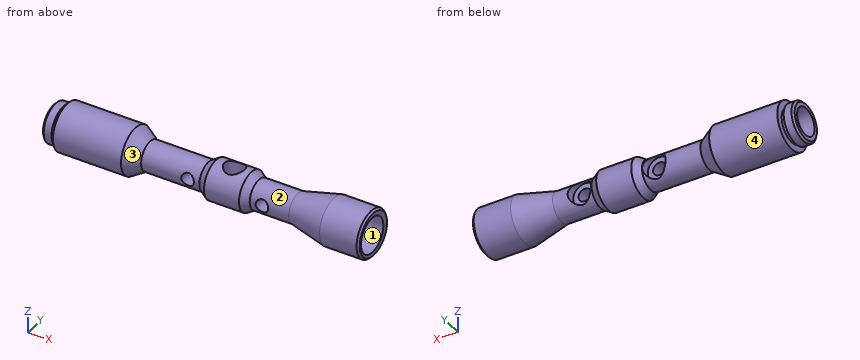
from build123d import *

# Parameters (mm, degrees)
HOLE_WIZARD_9_D            = 10
HOLE_WIZARD_9_DEPTH        = 50
HOLE_WIZARD_9_CBORE_D      = 14
HOLE_WIZARD_9_CBORE_DEPTH  = 20
HOLE_WIZARD_9_TIP          = 2.886751346
HOLE_WIZARD_M12_1_D        = 10.2
HOLE_WIZARD_M12_1_DEPTH    = 12
HOLE_WIZARD_M12_1_TIP      = 3.064389157
CHAMFER_1_SIZE             = 1
CHAMFER_2_SIZE             = 1
HOLE_WIZARD_12_D           = 10
HOLE_WIZARD_12_DEPTH       = 40
HOLE_WIZARD_12_CBORE_D     = 18
HOLE_WIZARD_12_CBORE_DEPTH = 20
HOLE_WIZARD_12_TIP         = 2.886751346
HOLE_WIZARD_14_D           = 6.5
HOLE_WIZARD_14_DEPTH       = 100
HOLE_WIZARD_14_CBORE_D     = 12
HOLE_WIZARD_14_CBORE_DEPTH = 4.5
HOLE_WIZARD_15_D           = 6.5
HOLE_WIZARD_15_DEPTH       = 100
HOLE_WIZARD_15_CBORE_D     = 12
HOLE_WIZARD_15_CBORE_DEPTH = 4.5


with BuildPart() as part:
    # 草图2 → 旋转2 (revolve)
    with BuildSketch(Plane.XY, mode=Mode.PRIVATE) as revolve_2_sk:
        Polygon((0, 10), (0, 0), (164, 0), (164, 12), (144, 12), (125.3, 7.582380862), (105.3, 7.582380862), (101.324359639, 10), (83.324359639, 10), (79.4, 7.5), (49.4, 7.5), (42, 12), (7, 12), (7, 8.5), (5, 8.5), (5, 10), align=None)
    revolve(revolve_2_sk.sketch.rotate(Axis((0, 0, 0), (1, 0, 0)), 180), axis=Axis((0, 0, 0), (1, 0, 0)))

    # 孔9
    with Locations(Plane.ZY):
        with Locations((0, 0)):
            CounterBoreHole(HOLE_WIZARD_9_D / 2, HOLE_WIZARD_9_CBORE_D / 2, HOLE_WIZARD_9_CBORE_DEPTH, depth=HOLE_WIZARD_9_DEPTH)
            with Locations((0, 0, -(HOLE_WIZARD_9_DEPTH + HOLE_WIZARD_9_TIP / 2))):  # 120° drill point
                Cone(0, HOLE_WIZARD_9_D / 2, HOLE_WIZARD_9_TIP, mode=Mode.SUBTRACT)

    # M12 螺纹孔1
    with Locations(Plane(origin=(92.712048687, 0.00356299, 9.999999365), x_dir=(0, 0.999999936526, -0.000356298984), z_dir=(0, 0.000356298984, 0.999999936526))):
        with Locations((0, 0)):
            Hole(HOLE_WIZARD_M12_1_D / 2, depth=HOLE_WIZARD_M12_1_DEPTH)
            with Locations((0, 0, -(HOLE_WIZARD_M12_1_DEPTH + HOLE_WIZARD_M12_1_TIP / 2))):  # 118° drill point
                Cone(0, HOLE_WIZARD_M12_1_D / 2, HOLE_WIZARD_M12_1_TIP, mode=Mode.SUBTRACT)

    # 倒角1
    chamfer_1_edges = [part.edges().sort_by_distance(p)[0] for p in [
        (164, 12, 0),
    ]]
    chamfer(chamfer_1_edges, length=CHAMFER_1_SIZE)

    # 倒角2
    chamfer_2_edges = [part.edges().sort_by_distance(p)[0] for p in [
        (0, 10, 0),
    ]]
    chamfer(chamfer_2_edges, length=CHAMFER_2_SIZE)

    # 孔12
    with Locations(Plane(origin=(164, 0, 0), x_dir=(0, 0, -1), z_dir=(1, 0, 0))):
        with Locations((-0.105297268, -0.976154466)):
            CounterBoreHole(HOLE_WIZARD_12_D / 2, HOLE_WIZARD_12_CBORE_D / 2, HOLE_WIZARD_12_CBORE_DEPTH, depth=HOLE_WIZARD_12_DEPTH)
            with Locations((0, 0, -(HOLE_WIZARD_12_DEPTH + HOLE_WIZARD_12_TIP / 2))):  # 120° drill point
                Cone(0, HOLE_WIZARD_12_D / 2, HOLE_WIZARD_12_TIP, mode=Mode.SUBTRACT)

    # 孔14
    with Locations(Plane(origin=(73.309592569, 7.499999992, 0.000348053), x_dir=(0, -4.6407092e-05, 0.999999998923), z_dir=(0, 0.999999998923, 4.6407092e-05))):
        with Locations((0, 0)):
            CounterBoreHole(HOLE_WIZARD_14_D / 2, HOLE_WIZARD_14_CBORE_D / 2, HOLE_WIZARD_14_CBORE_DEPTH, depth=HOLE_WIZARD_14_DEPTH)

    # 孔15
    with Locations(Plane(origin=(111.545186108, 7.582371257, 0.012068763), x_dir=(0, -0.001591685193, 0.999998733268), z_dir=(0, 0.999998733268, 0.001591685193))):
        with Locations((0, 0)):
            CounterBoreHole(HOLE_WIZARD_15_D / 2, HOLE_WIZARD_15_CBORE_D / 2, HOLE_WIZARD_15_CBORE_DEPTH, depth=HOLE_WIZARD_15_DEPTH)


solid = part.part
Build history of the part. All positions in model axes, mm. Face numbers are marked on the shaded views. A direction names the side the tool comes from. Coordinates: 2 decimals unless noted, no trailing zeros. Write each loop counter-clockwise with the first axis right and the second up, starting at its lowest first coordinate (ties: lowest second). Pieces come first, ordered by that corner, then holes. Notation, with made-up numbers: (-25.5, 54) -> (26.5, 54) arc R12 cw to (26.5, 77) -> close; hole circle Ø5 at (11.5, -35.75). An arc over 180 degrees is marked (long way). Use CSV: the item, a comma, the result in double quotes. Start each with the question number.
Q1. Pull direction X, two halves, no side cores. Call the marked faces 1 and 2: released by +X, released by -X, zero draft, split by the parting line, or undercut.
Q2. Cut at A-A, the plane x = 85. List the corners of the cut face in (y, z), then the cut area to 3 significant figures.
Q3. 3-axis set-ups, long thin cutter, end or side, ignore diameter. For the marked faces 3 and 4: which of +Z, -Z, +X, -X, +Y, -Y reach the whole face in a straight line?
Q4. Flat gauge pins, fed straight in: pin 1 Ø12 at (x, z) = (84.5, 0) entering from +Y; pin 2 Ø1.5 at (y, z) = (-3, -1.5) entering from +X; pin 3 Ø4 at (y, z) = (-1.5, -0.5) entering from +X; pin 4 Ø13 at (y, z) = (-0.98, 0.11) entering from -X. Where does each tip first touch, or does it go through?
Q5. Drill centre lines: probe 1 along Y at (x, z) = (97, 2); probe 2 along Z at (x, y) = (57.5, -0.5); probe 3 along X at (y, z) = (5.5, 0.75). Where is each one in solid material? Low to high.
Checked values:
1,face 1,"zero draft"
1,face 2,"undercut"
2,outline,"circle Ø20 at (0, 0)"
2,area,"314 mm²"
3,face 3,"none"
3,face 4,"+X, -X"
4,pin 1,"stops at y = 10"
4,pin 2,"stops at x = 123.04"
4,pin 3,"stops at x = 122.73"
4,pin 4,"stops at x = 0"
5,probe 1,"y = -9.8 to -2.76, 2.76 to 9.8"
5,probe 2,"z = -7.48 to 7.48"
5,probe 3,"x = 20 to 67.36, 79.26 to 105.59, 117.5 to 144"
